from build123d import *

# Parameters (mm, degrees)
F1_DEPTH = 16
F3_D     = 3.8
F3_DEPTH = 20
F3_TIP   = 1.1416351762
F4_SIZE  = 1.5


with BuildPart() as f1:
    # F0 (on Top) → F1 (new body)
    with BuildSketch(Plane.XY):
        with BuildLine():
            Line((-74, -14.8000685584), (-74, 61.1999314416))
            Line((-74, 61.1999314416), (-90, 61.1999314416))
            Line((-90, 61.1999314416), (-90, -14.8000685584))
            ThreePointArc((-90, -14.8000685584), (-74.5730833817, -42.1740143321), (-43.1666932985, -43.1544864205))
            ThreePointArc((-43.1666932985, -43.1544864205), (-22.2256381935, -35.236562411), (0, -32.5454071904))
            ThreePointArc((0, -32.5454071904), (22.2256381935, -35.236562411), (43.1666932985, -43.1544864205))
            ThreePointArc((43.1666932985, -43.1544864205), (74.5730833817, -42.1740143321), (90, -14.8000685584))
            Line((90, -14.8000685584), (90, 61.1999314416))
            Line((90, 61.1999314416), (74, 61.1999314416))
            Line((74, 61.1999314416), (74, -14.8000685584))
            ThreePointArc((74, -14.8000685584), (66.2865416908, -28.4870414452), (50.5833466493, -28.9772774894))
            ThreePointArc((50.5833466493, -28.9772774894), (26.0443197136, -19.6989412466), (0, -16.5454071904))
            ThreePointArc((0, -16.5454071904), (-26.0443197136, -19.6989412466), (-50.5833466493, -28.9772774894))
            ThreePointArc((-50.5833466493, -28.9772774894), (-66.2865416908, -28.4870414452), (-74, -14.8000685584))
        make_face()
    extrude(amount=F1_DEPTH)

    # F3
    with Locations(Plane(origin=(0, 61.1999314416, 0), x_dir=(-1, 0, 0), z_dir=(0, 1, 0))):
        with Locations((82, 8), (-82, 8)):
            Hole(F3_D / 2, depth=F3_DEPTH)
            with Locations((0, 0, -(F3_DEPTH + F3_TIP / 2))):  # 118° drill point
                Cone(0, F3_D / 2, F3_TIP, mode=Mode.SUBTRACT)

    # F4
    f4_edges = [f1.edges().sort_by_distance(p)[0] for p in [
        (74.573083, -42.174014, 0),
        (66.286542, -28.487041, 0),
    ]]
    chamfer(f4_edges, length=F4_SIZE)


solid = f1.part
Could you check a few things on this model? Use its own coordinates, in mm. A direction names the side the tool comes from. Give positions to 0.01 mm unless a question says otherwise; leave off trailing zeros. Order: outer loops, then holes, each group sorted by start corner. A loop starts at its lowest first (then second) coordinate and runs counter-clockwise, first axis right, second up. Notation, with made-up numbers: (30, -23) - (74, -23) arc R18 cw to (74, -19) - close; hole circle Ø10 at (28.5, 15). An arc over 180 degrees is marked (long way). One line per question, with ' | ' between items. Start each with the question number.
Item 1: I'm going to push flat-ended pins straight in: pin 1 Ø8 at (y, z) = (-19.5, 1.5) entering from +X; pin 2 Ø1 at (x, z) = (3, 13) entering from -Y; pin 3 Ø3 at (x, z) = (-14.5, 3.5) entering from -Y. Where does each tip first touch, or does it pass through?
Item 2: Thinking about a two-plate mould opening in Z: for faces 1 (the flat face through (-74, 23, 9)), 2 (the flat face through (-7, -19, 0)), 3 (the cylindrical face through (80.1, 51.06, 8.08)), which applies, pulls with the +Z half, pulls with the -Z half, needs draft (parallel to the pull), parting line crosses it, or undercut?
Item 3: I want a section at A-A on y = 44. Write out the boundary of the cut face in (x, z), then the cut area to 3 significant figures.
Item 4: I want a section at B-B on y = -7. Write out the boundary of the cut face in (x, z).
Item 5: For faces 4 (the flat face through (84, 61.2, 10)), 5 (the cylindrical face through (-83.9, 51.06, 8.08)), 6 (the flat face through (74, 24, 9)), which set-ups out of +Z, -Z, +X, -X, +Y, -Y let a thin tool reach every point of the face, with its end or its side?
Item 6: I need wall thicknesses on probe 1 along X at (y, z) = (46.5, 8); probe 2 along X at (y, z) = (42.5, 14.25); probe 3 along Z at (x, y) = (82, 51). Which ranges of each line are inside material? Lowest first, please. Write a range as [from, to].
Item 7: I want a section at C-C on z = 3.25. Write out the boundary of the cut face in (x, y).
Verdict:
1) pin 1: x = 89.99 | pin 2: y = -32.61 | pin 3: y = -33.93
2) face 1: needs draft | face 2: pulls with the -Z half | face 3: undercut
3) outline: (-90, 1.5) - (-88.5, 0) - (-75.5, 0) - (-74, 1.5) - (-74, 16) - (-90, 16) - close; (74, 1.5) - (75.5, 0) - (88.5, 0) - (90, 1.5) - (90, 16) - (74, 16) - close; hole circle Ø3.8 at (-82, 8); hole circle Ø3.8 at (82, 8) | area: 485 mm^2
4) outline: (-90, 1.5) - (-88.5, 0) - (-75.5, 0) - (-74, 1.5) - (-74, 16) - (-90, 16) - close; (74, 1.5) - (75.5, 0) - (88.5, 0) - (90, 1.5) - (90, 16) - (74, 16) - close
5) face 4: +Z, -Z, +X, -X, +Y | face 5: +Y | face 6: +Z, -Z, +Y
6) probe 1: [-90, -83.9], [-80.1, -74], [74, 80.1], [83.9, 90] | probe 2: [-90, -74], [74, 90] | probe 3: [0, 6.1], [9.9, 16]
7) outline: (-90, -14.8) arc R32 ccw to (-43.17, -43.15) arc R93.12 cw to (43.17, -43.15) arc R32 ccw to (90, -14.8) - (90, 61.2) - (74, 61.2) - (74, -14.8) arc R16 cw to (50.58, -28.98) arc R109.12 ccw to (-50.58, -28.98) arc R16 cw to (-74, -14.8) - (-74, 61.2) - (-90, 61.2) - close
